The model under review builds one solid part; all positions refer to its coordinate system, in mm. Face numbers are marked on the shaded views. A direction names the side the tool comes from. Round coordinates to 2 decimals unless told otherwise and drop trailing zeros. Loops run counter-clockwise (first coordinate to the right, second up) from the corner with the lowest first, then second, coordinate; pieces in that order, holes last. Notation, with made-up numbers: M 33.25,38 L 44.25,38 A38 ccw 44.25,76 Z; hole C -32.75,59 d10. An arc over 180 degrees is marked long. Return JSON: item names as keys, results as strings. Group by question number.
Q1. Draft analysis for pull direction Z (two halves, no side actions). For the marked faces 1, 2, 3 and 4, state which applies: pulls with the +Z half, pulls with the -Z half, needs draft (parallel to the pull), parting line crosses it, or undercut.
Q2. For the marked faces 5 and 6, list the 3-axis set-ups (+Z, -Z, +X, -X, +Y, -Y) from which the entire face can be reached by the end or side of a thin tool; tool diameter is ignored.
Q3. Consider section D-D (z = 10). State the section outline as (x, y) points, and give its area (3 significant figures).
Q4. Consider section A-A (x = -3.75). State the section outline as (y, z) points.
Q5. Consider section C-C (y = 0). Count the separate pieces of the cut face and the enclosed holes in it, and give its area (3 significant figures).
Q6. Consider section B-B (y = -8). State the section outline as (x, z) points, and give its area (3 significant figures).
Q7. Clearance check with flat-ended pins moving along their axes: pin 1 Ø3.5 at (x, y) = (-8, 13.5) entering from +Z; pin 2 Ø3.5 at (y, z) = (0, -48) entering from +X; pin 3 Ø1.5 at (y, z) = (-0.5, -48) entering from -X. State where each tip first meets the part, or that it passes through.
Q8. To check wall thickness, follow line 1 along Z through (x, y) = (-10, 7); line 2 along Z through (x, y) = (4, -8.5); line 3 along Y through (x, z) = (7.75, -2.1). State the ranges of each line that lie inside material, in increasing order.
from build123d import *

# Parameters (mm, degrees)
SKETCH_2_R          = 18.5
EXTRUDE_1_DEPTH     = 24
SKETCH_3_R          = 16
EXTRUDE_2_DEPTH     = 22
SKETCH_4_R          = 3
SKETCH_4_W          = 0.5
SKETCH_4_H          = 3
EXTRUDE_3_DEPTH     = 3
SKETCH_5_R          = 16.15
EXTRUDE_4_DEPTH     = 1
SKETCH_6_R          = 6.8
SKETCH_6_W          = 16
SKETCH_6_H          = 9.3
EXTRUDE_7_DEPTH     = 5
SKETCH_7_R          = 0.75
EXTRUDE_8_DEPTH     = 5
SKETCH_8_R          = 6
EXTRUDE_9_DEPTH     = 6
SKETCH_9_R          = 3
EXTRUDE_10_DEPTH    = 15
CUT_EXTRUDE_START   = -12
CUT_EXTRUDE_1_DEPTH = 12
SKETCH_11_R         = 1.5
CUT_EXTRUDE_2_DEPTH = 3.5


with BuildPart() as part:
    # 스케치2 → 보스-돌출1 (new body)
    with BuildSketch(Plane.XY):
        Circle(SKETCH_2_R)
    extrude(amount=-EXTRUDE_1_DEPTH)

    # 스케치3 → 보스-돌출2 (add)
    with BuildSketch(Plane(origin=(0, 0, -24), x_dir=(-1, 0, 0), z_dir=(0, 0, -1))):
        Circle(SKETCH_3_R)
    extrude(amount=EXTRUDE_2_DEPTH)

    # 스케치4 → 보스-돌출3 (add)
    with BuildSketch(Plane(origin=(0, 0, -46), x_dir=(-1, 0, 0), z_dir=(0, 0, -1))):
        Circle(SKETCH_4_R)
        with Locations((14, 0)):
            Rectangle(SKETCH_4_W, SKETCH_4_H)
        with Locations((-14, 0)):
            Rectangle(SKETCH_4_W, SKETCH_4_H)
    extrude(amount=EXTRUDE_3_DEPTH)

    # 스케치5 → 보스-돌출4 (add)
    with BuildSketch(Plane(origin=(0, 0, -49), x_dir=(-1, 0, 0), z_dir=(0, 0, -1))):
        Circle(SKETCH_5_R)
    extrude(amount=EXTRUDE_4_DEPTH)

    # 스케치6 → 보스-돌출7 (add)
    with BuildSketch(Plane(origin=(0, 0, -50), x_dir=(-1, 0, 0), z_dir=(0, 0, -1))):
        Circle(SKETCH_6_R)
        with Locations((0, -11.5)):
            Rectangle(SKETCH_6_W, SKETCH_6_H)
    extrude(amount=EXTRUDE_7_DEPTH)

    # 스케치7 → 보스-돌출8 (add)
    with BuildSketch(Plane.XZ.offset(16.15)):
        with Locations(Location((-6.25, -52.5, 0), (0, 0, 90))):
            Circle(SKETCH_7_R)
        with Locations(Location((-3.75, -52.5, 0), (0, 0, 90))):
            Circle(SKETCH_7_R)
        with Locations(Location((-1.25, -52.5, 0), (0, 0, 90))):
            Circle(SKETCH_7_R)
        with Locations(Location((1.25, -52.5, 0), (0, 0, 90))):
            Circle(SKETCH_7_R)
        with Locations(Location((3.75, -52.5, 0), (0, 0, 90))):
            Circle(SKETCH_7_R)
        with Locations(Location((6.25, -52.5, 0), (0, 0, 90))):
            Circle(SKETCH_7_R)
    extrude(amount=EXTRUDE_8_DEPTH)

    # 스케치8 → 보스-돌출9 (add)
    with BuildSketch(Plane.XY):
        with Locations((0, 7.5)):
            Circle(SKETCH_8_R)
    extrude(amount=EXTRUDE_9_DEPTH)

    # 스케치9 → 보스-돌출10 (add)
    with BuildSketch(Plane.XY.offset(6)):
        with Locations((0, 7.5)):
            Circle(SKETCH_9_R)
    extrude(amount=EXTRUDE_10_DEPTH)

    # 스케치10 → 컷-돌출1 (cut)
    with BuildSketch(Plane.XY.offset(21).offset(CUT_EXTRUDE_START)):
        with BuildLine():
            Line((-1.658312395, 10), (1.658312395, 10))
            ThreePointArc((1.658312395, 10), (0, 10.5), (-1.658312395, 10))
        make_face()
    extrude(amount=CUT_EXTRUDE_1_DEPTH, mode=Mode.SUBTRACT)

    # 스케치11 → 컷-돌출2 (cut)
    with BuildSketch(Plane.XY):
        with Locations((15.5, 0)):
            Circle(SKETCH_11_R)
        with Locations((7.75, -13.423393759)):
            Circle(SKETCH_11_R)
        with Locations((-7.75, -13.423393759)):
            Circle(SKETCH_11_R)
        with Locations((-15.5, 0)):
            Circle(SKETCH_11_R)
        with Locations((-7.75, 13.423393759)):
            Circle(SKETCH_11_R)
        with Locations((7.75, 13.423393759)):
            Circle(SKETCH_11_R)
    extrude(amount=-CUT_EXTRUDE_2_DEPTH, mode=Mode.SUBTRACT)


solid = part.part
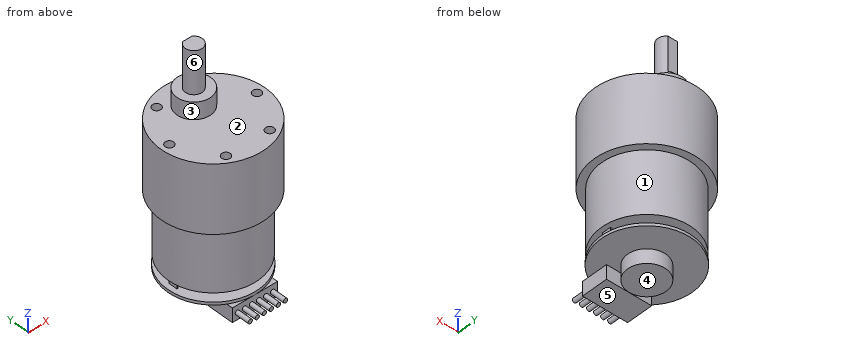
Values:
{
 "1": {"face 1": "undercut", "face 2": "pulls with the +Z half", "face 3": "needs draft", "face 4": "pulls with the -Z half"},
 "2": {"face 5": "-Z, +X, -X, +Y, -Y", "face 6": "+Z"},
 "3": {"outline": "M -1.66,10 A3 ccw long 1.66,10 Z", "area": "27.1 mm2"},
 "4": {"outline": "M -21.15,-53.25 L -16.15,-53.25 L -16.15,-55 L -6.85,-55 L -6.85,-50 L -5.67,-50 L -5.67,-55 L 5.67,-55 L 5.67,-50 L 15.71,-50 L 15.71,-49 L -15.71,-49 L -15.71,-50 L -16.15,-50 L -16.15,-51.75 L -21.15,-51.75 Z; M -18.12,-24 L -15.55,-24 L -15.55,-46 L 15.55,-46 L 15.55,-24 L 18.12,-24 L 18.12,0 L 12.18,0 L 12.18,6 L 2.82,6 L 2.82,0 L -18.12,0 Z"},
 "5": {"separate pieces": "1", "enclosed holes": "2", "area": "1,690 mm2"},
 "6": {"outline": "M -16.68,-24 L -13.86,-24 L -13.86,-46 L 13.86,-46 L 13.86,-24 L 16.68,-24 L 16.68,0 L -16.68,0 Z; M -14.03,-50 L -8,-50 L -8,-55 L 8,-55 L 8,-50 L 14.03,-50 L 14.03,-49 L -14.03,-49 Z", "area": "1,520 mm2"},
 "7": {"pin 1": "stops at z = 0", "pin 2": "stops at x = 16.15", "pin 3": "stops at x = -14.25"},
 "8": {"line 1": "z = -50 to -49, -46 to 0", "line 2": "z = -55 to -49, -46 to 0", "line 3": "y = -16.8 to -14.92, -11.92 to 11.92, 14.92 to 16.8"}
}
